```python
from build123d import *

# Parameters (mm, degrees)
F0_R     = 7.5
F0_R_2   = 7.25
F0_R_3   = 6
F1_DEPTH = 16
F2_DEPTH = 12
F3_DEPTH = 1.5


with BuildPart() as f1:
    # F0 (on Top) → F1 (new body)
    with BuildSketch(Plane.XY):
        Circle(F0_R)
        Circle(F0_R_2, mode=Mode.SUBTRACT)
        Circle(F0_R_2)
        Circle(F0_R_3, mode=Mode.SUBTRACT)
        Circle(F0_R_3)
    extrude(amount=-F1_DEPTH)

    # F0 (on Top) → F2 (cut)
    with BuildSketch(Plane.XY):
        Circle(F0_R_2)
        Circle(F0_R_3, mode=Mode.SUBTRACT)
    extrude(amount=-F2_DEPTH, mode=Mode.SUBTRACT)

    # F0 (on Top) → F3 (cut)
    with BuildSketch(Plane.XY):
        Circle(F0_R_3)
    extrude(amount=-F3_DEPTH, mode=Mode.SUBTRACT)


solid = f1.part
```
The listing builds one solid part. Answer for the finished solid, in the listing's coordinates (mm). Round coordinates to 2 decimals unless told otherwise and drop trailing zeros. Loops run counter-clockwise (first coordinate to the right, second up) from the corner with the lowest first, then second, coordinate; pieces in that order, holes last.
Q1. Find the intervals of material crossed by line 1 (X direction, y = -0.25, z = -7.75); line 2 (Y direction, x = 0, z = -4); line 3 (X direction, y = -2.5, z = -7.5), in increasing order.
Q2. For a pull along X with two mould halves and no side action, classify faces 1 (the face through (0, 0, -16)), 2 (the face through (0, 0, -1.5)), 3 (the face through (-7.493, 0.33, -7.888)) as released by +X, released by -X, zero draft, split by the parting line, or undercut.
Q3. Section A-A, the plane y = 0 is taken. Determine the outline of the cut face in (x, z).
Q4. Section D-D, the plane z = -13.5 is taken. Determine the outline of the cut face in (x, y).
Q5. Section C-C, the plane z = -8.25 is taken. Determine the outline of the cut face in (x, y), then the cut area to 3 significant figures.
Q6. Given pin 1 Ø1 at (x, z) = (4.5, -6.5) entering from +Y; pin 2 Ø5 at (y, z) = (-5, -13.5) entering from +X; pin 3 Ø7 at (x, y) = (2, -2.5) entering from +Z, each flat-ended and moving along its own axis, determine where each tip first touches the part or whether it passes through.
Completed:
1. line 1: x = -7.5 to -7.25, -5.99 to 5.99, 7.25 to 7.5
1. line 2: y = -7.5 to -7.25, -6 to 6, 7.25 to 7.5
1. line 3: x = -7.07 to -6.81, -5.45 to 5.45, 6.81 to 7.07
2. face 1: zero draft
2. face 2: undercut
2. face 3: split by the parting line
3. outline: (-7.5, -16) - (7.5, -16) - (7.5, 0) - (7.25, 0) - (7.25, -12) - (6, -12) - (6, -1.5) - (-6, -1.5) - (-6, -12) - (-7.25, -12) - (-7.25, 0) - (-7.5, 0) - close
4. outline: circle Ø15 at (0, 0)
5. outline: circle Ø15 at (0, 0); circle Ø12 at (0, 0); hole circle Ø14.5 at (0, 0)
5. area: 125 mm2
6. pin 1: stops at y = 6.34
6. pin 2: stops at x = 7.07
6. pin 3: stops at z = -1.5
